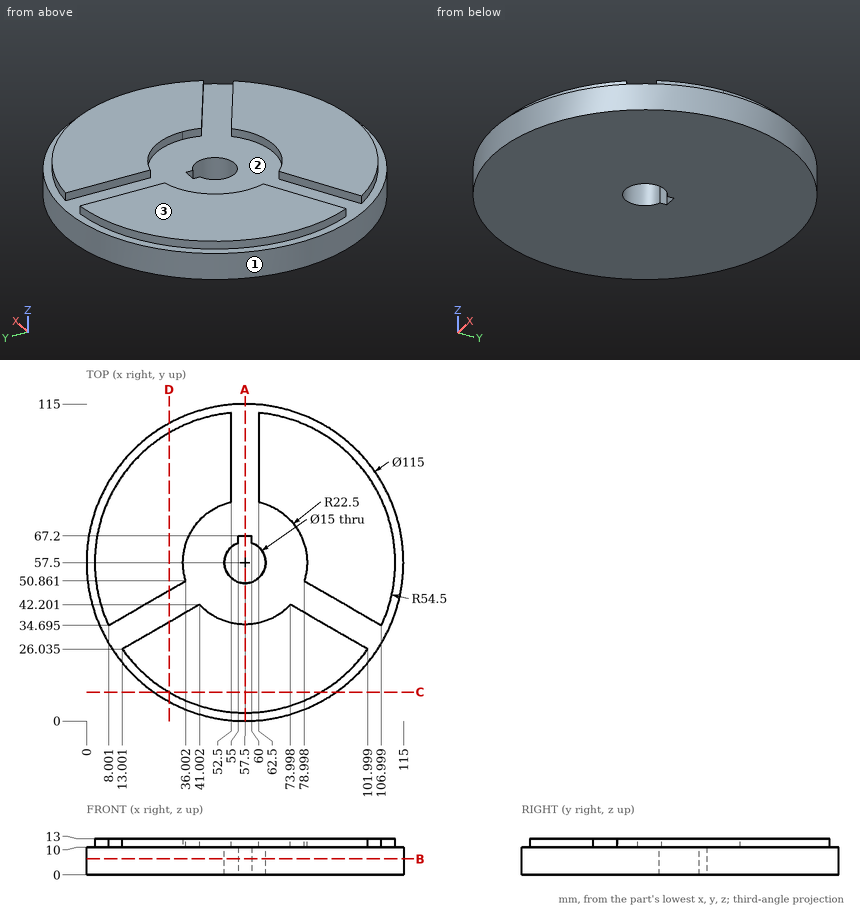
Design review of the part shown in the three views and the two pictorial views. Dimensions are in mm from the part's minimum x, y and z. Give positions to 0.01 mm unless a question says otherwise; leave off trailing zeros. Loops run counter-clockwise (first coordinate to the right, second up) from the corner with the lowest first, then second, coordinate; pieces in that order, holes last. Notation, with made-up numbers: (-6, 38) - (27, 38) arc R19 ccw to (27, 62) - close; hole circle Ø8 at (63, 20). An arc over 180 degrees is marked (long way). Use CSV: the item, a comma, the result in double quotes. Start each with the question number.
1. Add section C-C (y = 10.5). State the section outline as (x, z) points (1 decimal), plus the area to 3 significant figures.
2. Wall thickness on L1, parallel to Y at x = 57.5, z = 6; L2, parallel to Z at x = 62, y = 76; L3, parallel to Y at x = 95, z = 12.5 (1 decimal): over which ranges is each line inside the solid? List them lowest first.
3. Add section A-A (x = 57.5). State the section outline as (y, z) points.
4. Add section D-D (x = 30). State the section outline as (y, z) points, plus the area to 3 significant figures.
5. Add section B-B (z = 5.75). State the section outline as (x, y) points.
6. Insertion check: P1, Ø24, axis at x = 57.5, y = 57.5, coming from the +Z side; P2, Ø2.5, axis at y = 92, z = 12, coming from the -X side; P3, Ø1, axis at x = 27, z = 11, coming from the +Y side. Each pin has a flat end and moves straight along its axis. Give the tip position at first contact, or say it passes through.
7. Draft analysis for pull direction Y (two halves, no side actions). For the marked faces 1, 2 and 3, state which applies: released by +Y, released by -Y, zero draft, split by the parting line, or undercut.
Results found:
1,outline,"(24.4, 0) - (90.6, 0) - (90.6, 10) - (85.1, 10) - (85.1, 13) - (29.9, 13) - (29.9, 10) - (24.4, 10) - close"
1,area,"828 mm²"
2,L1,"y = 0 to 50, 67.2 to 115"
2,L2,"z = 0 to 10"
2,L3,"y = 18 to 30.1, 41.6 to 97"
3,outline,"(0, 0) - (50, 0) - (50, 10) - (35, 10) - (35, 13) - (3, 13) - (3, 10) - (0, 10) - close; (67.2, 0) - (115, 0) - (115, 10) - (67.2, 10) - close"
4,outline,"(7, 0) - (108, 0) - (108, 10) - (104.55, 10) - (104.55, 13) - (47.4, 13) - (47.4, 10) - (35.85, 10) - (35.85, 13) - (10.45, 13) - (10.45, 10) - (7, 10) - close"
4,area,"1,260 mm²"
5,outline,"circle Ø115 at (57.5, 57.5); hole (55, 64.57) arc R7.5 ccw (long way) to (60, 64.57) - (60, 67.2) - (55, 67.2) - close"
6,P1,"stops at z = 10"
6,P2,"stops at x = 14.32"
6,P3,"stops at y = 103"
7,face 1,"split by the parting line"
7,face 2,"undercut"
7,face 3,"zero draft"
